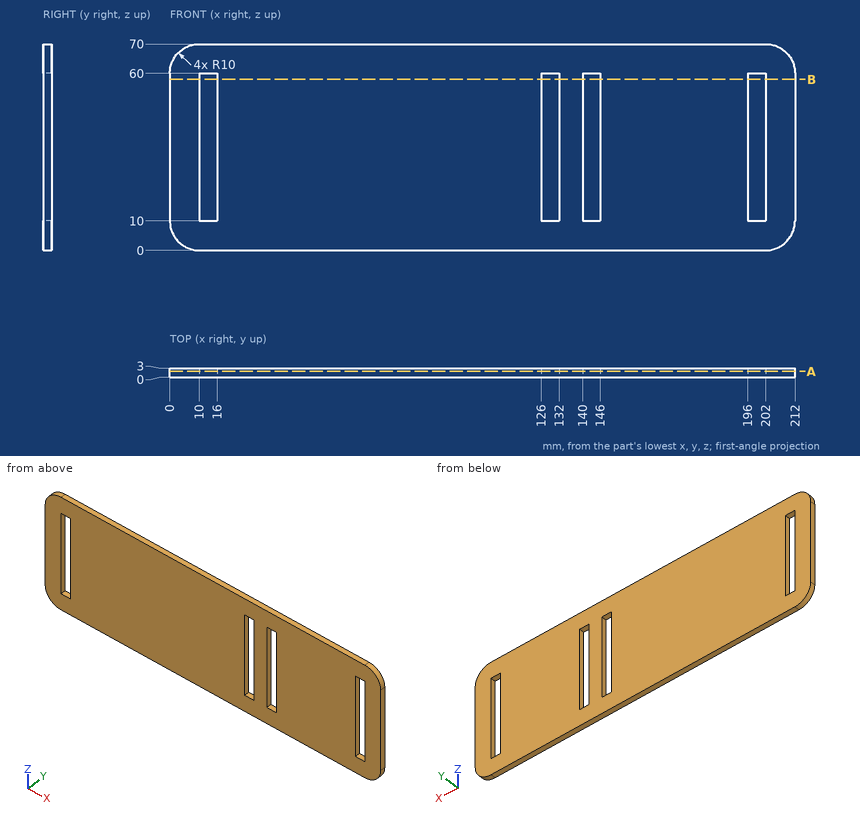
Input: dimensioned drawing with shaded views. Units: mm. Origin: part minimum x, y, z. Coordinates: 2 decimals unless noted, no trailing zeros. Loops run counter-clockwise (first coordinate to the right, second up) from the corner with the lowest first, then second, coordinate; pieces in that order, holes last. Notation, with made-up numbers: M 85.25,32.25 L 94.25,32.25 A29 ccw 94.25,71.25 Z; hole C -9,2.25 d9. An arc over 180 degrees is marked long. Use a Markdown table: item, result. Add a question column.
1) Pin query (flat end, axial travel): P1, Ø2, axis at x = 134, z = 45, coming from the -Y side. Return the tip coordinate at first contact, or that it passes through.
2) Section B-B, the plane z = 58. Return the cut outline in (x, y), plus the area to 3 significant figures.
3) Line query: L1, parallel to X at y = 1.55, z = 45.5; L2, parallel to Z at x = 141.5, y = 0.45; L3, parallel to X at y = 0.1, z = 62. Output: solid intervals per line, ascending. Write a range as from..to.
4) Section A-A, the plane y = 2. Return the cut outline in (x, z).
Answer below:
| question | item | result |
|---|---|---|
| 1 | P1 | y = 0 |
| 2 | outline | M 0,0 L 10,0 L 10,3 L 0,3 Z; M 16,0 L 126,0 L 126,3 L 16,3 Z; M 132,0 L 140,0 L 140,3 L 132,3 Z; M 146,0 L 196,0 L 196,3 L 146,3 Z; M 202,0 L 212,0 L 212,3 L 202,3 Z |
| 2 | area | 564 mm2 |
| 3 | L1 | 0..10, 16..126, 132..140, 146..196, 202..212 |
| 3 | L2 | 0..10, 60..70 |
| 3 | L3 | 0.2..211.8 |
| 4 | outline | M 0,10 A10 ccw 10,0 L 202,0 A10 ccw 212,10 L 212,60 A10 ccw 202,70 L 10,70 A10 ccw 0,60 Z; hole M 10,10 L 16,10 L 16,60 L 10,60 Z; hole M 126,10 L 132,10 L 132,60 L 126,60 Z; hole M 140,10 L 146,10 L 146,60 L 140,60 Z; hole M 196,10 L 202,10 L 202,60 L 196,60 Z |
